Build history of the part. All positions in model axes, mm. A direction names the side the tool comes from. Give positions to 0.01 mm unless a question says otherwise; leave off trailing zeros. Write each loop counter-clockwise with the first axis right and the second up, starting at its lowest first coordinate (ties: lowest second). Pieces come first, ordered by that corner, then holes. Notation, with made-up numbers: M -14.5,45.5 L 33.5,45.5 A12 cw 33.5,60.5 Z; hole C -29.75,86 d1. An arc over 180 degrees is marked long. Return JSON: item names as keys, results as strings. Group by question number.
Q1. Band-saw the part on B-B, the plane z = 0. Give the cut face in (x, y).
Q2. Wall check: probe 1 along X at (y, z) = (78.5, 30); probe 2 along X at (y, z) = (13, 4.5); probe 3 along Z at (x, y) = (-30.5, 90). Give the ranges that are in metal, low to high.
Q3. Pull direction X, two halves, no side cores. Call faces 1 (the flat face through (35, 50, 30)), 2 (the flat face through (0, 85, 46)), 3 (the cylindrical face through (35.38, 49.3, -32.44)): +X half, -X half, draft (parallel to the pull), parting line (faces both ways), or undercut.
Q4. Flat gauge pins, fed straight in: pin 1 Ø1 at (x, y) = (25, 18) entering from -Z; pin 2 Ø10 at (y, z) = (84.5, -15) entering from -X; pin 3 Ø1.5 at (x, y) = (10.5, 84.5) entering from -Z. Where does each tip first touch, or does it go through?
Q5. Tool access for faces 4 (the flat face through (-14, 100, 43)), 5 (the cylindrical face through (-39.094, 19.355, -25.568)), 6 (the cylindrical face through (-25.568, 19.355, 39.094)): list every direction of +Z, -Z, +X, -X, +Y, -Y with a clear straight run to the whole face (end or side of a thin tool).
Q6. Band-saw the part on A-A, the plane x = 0. Give the cut face in (y, z).
Q7. Band-saw the part on C-C, the plane y = 87. Give the cut face in (x, z).
Autodesk Inventor part; units mm, degrees
ref_plane "YZ Plane" through (0, 0, 0) normal (1, 0, 0) x (0, 1, 0)
ref_plane "XZ Plane" through (0, 0, 0) normal (0, 1, 0) x (-1, 0, 0)
ref_plane "XY Plane" through (0, 0, 0) normal (0, 0, 1) x (1, 0, 0)
sketch "Sketch1" plane through (0, 0, 0) normal (0, 1, 0) x (-1, 0, 0)
  circle A0 centre (0, 0) radius 48
  dimension "d0" = 96
extrude "Extrusion1" add sketch "Sketch1" along normal blind 100
sketch "Sketch2" plane through (0, 100, 0) normal (0, 1, 0) x (1, 0, 0)
  circle A0 centre (0, 0) radius 45
  dimension "d3" = 90
extrude "Extrusion2" cut sketch "Sketch2" against normal blind 100
sketch "Sketch3" plane through (0, 0, 0) normal (0, 0, 1) x (1, 0, 0)
  line L0 (-15, 85) -> (15, 85)
  line L1 (30, 70) -> (30, 30)
  line L2 (15, 15) -> (-15, 15)
  line L3 (-30, 30) -> (-30, 70)
  line L4 (-30, 85) -> (30, 15) construction
  line L5 (30, 85) -> (-30, 15) construction
  arc A0 (30, 70) -> (15, 85) centre (15, 70) ccw
  arc A1 (-15, 85) -> (-30, 70) centre (-15, 70) ccw
  arc A2 (-30, 30) -> (-15, 15) centre (-15, 30) ccw
  arc A3 (15, 15) -> (30, 30) centre (15, 30) ccw
  point P0 (0, 0)
  point P1 (0, 50)
  dimension "d6" = 60
  dimension "d7" = 70
  dimension "d8" = 15
extrude "Extrusion3" cut sketch "Sketch3" along normal blind 100
pattern_circular "Circular Pattern1" count 4 over 360 about axis through (0, 100, 0) along (0, -1, 0) of "Extrusion3"
properties part number "Khay đựng cốc"
From the geometry:
{
 "1": {"outline": "M -48,0 L -45,0 L -45,15 L -48,15 Z; M -48,85 L -45,85 L -45,100 L -48,100 Z; M 45,0 L 48,0 L 48,15 L 45,15 Z; M 45,85 L 48,85 L 48,100 L 45,100 Z"},
 "2": {"probe 1": "x = -37.47 to -33.54, 33.54 to 37.47", "probe 2": "x = -47.79 to -44.77, 44.77 to 47.79", "probe 3": "z = -37.06 to -33.09, 33.09 to 37.06"},
 "3": {"face 1": "draft", "face 2": "undercut", "face 3": "parting line"},
 "4": {"pin 1": "stops at z = -41.28", "pin 2": "stops at x = -46.94", "pin 3": "stops at z = -46.96"},
 "5": {"face 4": "+Z, -Z, +X, -X, +Y", "face 5": "+X, -X", "face 6": "+Z, -Z"},
 "6": {"outline": "M 0,-48 L 15,-48 L 15,-45 L 0,-45 Z; M 0,45 L 15,45 L 15,48 L 0,48 Z; M 85,-48 L 100,-48 L 100,-45 L 85,-45 Z; M 85,45 L 100,45 L 100,48 L 85,48 Z"},
 "7": {"outline": "C 0,0 d96; hole C 0,0 d90"}
}
